Geometry check sheet. Reference: the model listing, model coordinates, mm. Coordinates: 2 decimals unless noted, no trailing zeros. Write each loop counter-clockwise with the first axis right and the second up, starting at its lowest first coordinate (ties: lowest second). Pieces come first, ordered by that corner, then holes. Notation, with made-up numbers: M 33,-17 L 48,-17 A25 ccw 48,12 Z; hole C -9,33 d10. An arc over 180 degrees is marked long. Write each question's results on one line, items separated by ' | '.
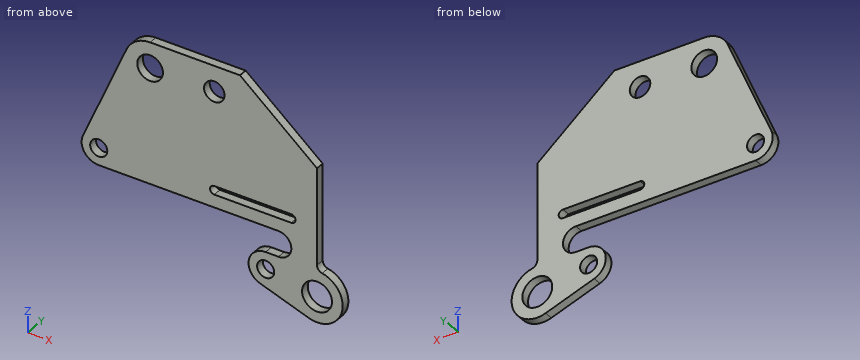
```python
from build123d import *

# Parameters (mm, degrees)
SKETCH1_R           = 25.4
SKETCH1_R_2         = 38.1
SKETCH1_R_3         = 44.45
SKETCH1_R_4         = 30.48
BOSS_EXTRUDE1_DEPTH = 12.7


with BuildPart() as part:
    # Sketch1 → Boss-Extrude1 (new body, symmetric)
    with BuildSketch(Plane(origin=(0, 0, 0), x_dir=(1, 0, 0), z_dir=(0, 1, 0))):
        with BuildLine():
            Line((-199.116056599, 272.143796557), (-70.074084898, -29.934305164))
            ThreePointArc((-70.074084898, -29.934305164), (-41.984794548, -63.590227447), (0, -76.2))
            Line((0, -76.2), (266.7, -76.2))
            Line((266.7, -76.2), (495.3, 115.618175687))
            Line((495.3, 115.618175687), (495.3, 401.9744408))
            ThreePointArc((495.3, 401.9744408), (499.593933451, 414.022718685), (510.54, 420.63955264))
            ThreePointArc((510.54, 420.63955264), (568.823505812, 515.318343915), (470.586486486, 567.381081081))
            Line((470.586486486, 567.381081081), (326.424324324, 517.954054054))
            ThreePointArc((326.424324324, 517.954054054), (292.791188669, 461.548531445), (342.9, 419.1))
            Line((342.9, 419.1), (381, 419.1))
            ThreePointArc((381, 419.1), (419.1, 381), (381, 342.9))
            Line((381, 342.9), (-152.4, 342.9))
            ThreePointArc((-152.4, 342.9), (-194.793484965, 320.089863032), (-199.116056599, 272.143796557))
        make_face()
        with Locations((-152.4, 292.1)):
            Circle(SKETCH1_R, mode=Mode.SUBTRACT)
        Circle(SKETCH1_R_2, mode=Mode.SUBTRACT)
        with Locations((342.9, 469.9)):
            Circle(SKETCH1_R, mode=Mode.SUBTRACT)
        with Locations((495.3, 495.3)):
            Circle(SKETCH1_R_3, mode=Mode.SUBTRACT)
        with Locations((190.5, 0)):
            Circle(SKETCH1_R_4, mode=Mode.SUBTRACT)
        with BuildLine():
            Line((190.5, 304.8), (419.1, 304.8))
            ThreePointArc((419.1, 304.8), (431.8, 292.1), (419.1, 279.4))
            Line((419.1, 279.4), (190.5, 279.4))
            ThreePointArc((190.5, 279.4), (177.8, 292.1), (190.5, 304.8))
        make_face(mode=Mode.SUBTRACT)
    extrude(amount=BOSS_EXTRUDE1_DEPTH, both=True)


solid = part.part
```
Q1. Sectioned sample at A-A on x = 233.5. Record the cut outline in (y, z), and give its area (4 significant figures).
Geometry check:
outline: M -12.7,-342.9 L 12.7,-342.9 L 12.7,-304.8 L -12.7,-304.8 Z; M -12.7,-279.4 L 12.7,-279.4 L 12.7,76.2 L -12.7,76.2 Z | area: 10,000 mm2
Q2. Scan lines: probe 1 along Z at (x, y) = (190.5, 4.5); probe 2 along Z at (x, y) = (364, 9.5); probe 3 along X at (y, z) = (-2.75, 0). Record each from-to range of solid material in increasing order.
Geometry check:
probe 1: z = -342.9 to -304.8, -279.4 to -30.48, 30.48 to 76.2 | probe 2: z = -530.84 to -484.04, -455.76 to -419.1, -342.9 to -304.8, -279.4 to -5.44 | probe 3: x = -82.86 to -38.1, 38.1 to 160.02, 220.98 to 357.51
Q3. Sectioned sample at D-D on x = 401.5. Record the cut outline in (y, z), and give its area (3 significant figures).
Geometry check:
outline: M -12.7,-543.69 L 12.7,-543.69 L 12.7,-413.11 L -12.7,-413.11 Z; M -12.7,-348.89 L 12.7,-348.89 L 12.7,-304.8 L -12.7,-304.8 Z; M -12.7,-279.4 L 12.7,-279.4 L 12.7,-36.91 L -12.7,-36.91 Z | area: 10,600 mm2
Q4. Sectioned sample at B-B on y = 2. Record the cut outline in (x, z).
Geometry check:
outline: M -199.12,-272.14 A50.8 ccw -152.4,-342.9 L 381,-342.9 A38.1 cw 381,-419.1 L 342.9,-419.1 A50.8 ccw 326.42,-517.95 L 470.59,-567.38 A76.2 ccw long 510.54,-420.64 A19.05 cw 495.3,-401.97 L 495.3,-115.62 L 266.7,76.2 L 0,76.2 A76.2 ccw -70.07,29.93 Z; hole C -152.4,-292.1 d50.8; hole C 0,0 d76.2; hole C 190.5,0 d60.96; hole M 190.5,-304.8 L 419.1,-304.8 A12.7 ccw 419.1,-279.4 L 190.5,-279.4 A12.7 ccw Z; hole C 342.9,-469.9 d50.8; hole C 495.3,-495.3 d88.9
Q5. Sectioned sample at C-C on z = 15.5. Record the cut outline in (x, y), and give its area (3 significant figures).
Geometry check:
outline: M -76.24,-12.7 L -34.8,-12.7 L -34.8,12.7 L -76.24,12.7 Z; M 34.8,-12.7 L 164.26,-12.7 L 164.26,12.7 L 34.8,12.7 Z; M 216.74,-12.7 L 339.04,-12.7 L 339.04,12.7 L 216.74,12.7 Z | area: 7,450 mm2
Q6. Depth check by flat-ended pin: P1, Ø5, axis at x = 145.5, y = 0, coming from the -Z side; P2, Ø7.5, axis at x = 345.5, y = -6, coming from the +Z side; P3, Ø6, axis at x = 361.5, y = 3, coming from the -Z side. Enter the tip coordinate at first touch or a pass-through.
Geometry check:
P1: stops at z = -342.9 | P2: stops at z = 13.23 | P3: stops at z = -531.01
